Design review of the part built by this model. Coordinates are the model's own, in mm. A direction names the side the tool comes from. Round coordinates to 2 decimals unless told otherwise and drop trailing zeros. Order: outer loops, then holes, each group sorted by start corner. A loop starts at its lowest first (then second) coordinate and runs counter-clockwise, first axis right, second up. Notation, with made-up numbers: (36, 25) - (51, 25) arc R25 cw to (51, 49) - close; hole circle Ø9 at (56.25, 50.5). An arc over 180 degrees is marked (long way). Answer as a JSON object with one key per item and string values. Group by question number.
from build123d import *

# Parameters (mm, degrees)
MODEL_R             = 8
BOSS_EXTRUDE1_DEPTH = 3


with BuildPart() as part:
    # Model → Boss-Extrude1 (new body)
    with BuildSketch(Plane.XY):
        Polygon((11.949818483, 0.880696589), (11.949818483, 30.880698285), (22.949818483, 30.884397455), (22.949818483, 33.884397625), (49.949818483, 33.893477406), (49.949818483, 30.893477236), (60.949818483, 30.897176406), (60.949818483, 0.89717471), (49.949818483, 0.89347554), (49.949818483, -2.10652463), (22.949818483, -2.115604411), (22.949818483, 0.884395759), align=None)
        with Locations((22.949818483, 13.879651404)):
            Circle(MODEL_R, mode=Mode.SUBTRACT)
        with Locations((49.949818483, 13.879651404)):
            Circle(MODEL_R, mode=Mode.SUBTRACT)
    extrude(amount=BOSS_EXTRUDE1_DEPTH)


solid = part.part
1. Mouldability with a two-part tool opening along Y and no side actions: class faces 1 (the cylindrical face through (21.91, 21.81, 1.48)), 2 (the flat face through (11.95, 16, 1)) as pulls with the +Y half, pulls with the -Y half, needs draft (parallel to the pull), parting line crosses it, or undercut.
2. To check wall thickness, follow line 1 (X direction, y = 11.5, z = 1.55); line 2 (X direction, y = 9, z = 0.75); line 3 (Y direction, x = 44, z = 2.25). State the ranges of each line that lie inside material, in increasing order. Write a range as from..to.
3. Take a section at D-D, the plane x = 19. Give the boundary of the cut face in (y, z).
4. Take a section at B-B, the plane x = 51. Give the boundary of the cut face in (y, z), then the cut area to 3 significant figures.
5. Clearance check with flat-ended pins moving along their axes: P1, Ø1, axis at x = 35.5, z = 1, coming from the -Y side; P2, Ø0.9, axis at x = 15, z = 2, coming from the -Y side; P3, Ø1.5, axis at x = 15.5, z = 2, coming from the +Y side. State where each tip first meets the part, or that it passes through.
6. Tool access review of faces 3 (the flat face through (22.95, 32, 1)), 4 (the flat face through (22.95, -1, 1)), 5 (the flat face through (49.95, -1, 1)), 6 (the flat face through (37, 16, 0)), 7 (the flat face through (49.95, 32, 1)): name each direction out of +Z, -Z, +X, -X, +Y, -Y from which nothing blocks a thin tool from reaching the whole face with its end or side.
7. Take a section at A-A, the plane y = 11. Give the boundary of the cut face in (x, z), then the cut area to 3 significant figures.
8. Take a section at C-C, the plane z = 2.1. Give the boundary of the cut face in (x, y).
Response values:
{
 "1": {"face 1": "undercut", "face 2": "needs draft"},
 "2": {"line 1": "11.95..15.31, 30.59..42.31, 57.59..60.95", "line 2": "11.95..16.61, 29.29..43.61, 56.29..60.95", "line 3": "-2.11..8.53, 19.23..33.89"},
 "3": {"outline": "(0.88, 0) - (6.92, 0) - (6.92, 3) - (0.88, 3) - close; (20.84, 0) - (30.88, 0) - (30.88, 3) - (20.84, 3) - close"},
 "4": {"outline": "(0.89, 0) - (5.95, 0) - (5.95, 3) - (0.89, 3) - close; (21.81, 0) - (30.89, 0) - (30.89, 3) - (21.81, 3) - close", "area": "42.4 mm2"},
 "5": {"P1": "y = -2.11", "P2": "y = 0.88", "P3": "y = 30.88"},
 "6": {"face 3": "+Z, -Z, -X, +Y", "face 4": "+Z, -Z, -X, -Y", "face 5": "+Z, -Z, +X, -Y", "face 6": "-Z, +X, -X, +Y, -Y", "face 7": "+Z, -Z, +X, +Y"},
 "7": {"outline": "(11.95, 0) - (15.49, 0) - (15.49, 3) - (11.95, 3) - close; (30.41, 0) - (42.49, 0) - (42.49, 3) - (30.41, 3) - close; (57.41, 0) - (60.95, 0) - (60.95, 3) - (57.41, 3) - close", "area": "57.4 mm2"},
 "8": {"outline": "(11.95, 0.88) - (22.95, 0.88) - (22.95, -2.12) - (49.95, -2.11) - (49.95, 0.89) - (60.95, 0.9) - (60.95, 30.9) - (49.95, 30.89) - (49.95, 33.89) - (22.95, 33.88) - (22.95, 30.88) - (11.95, 30.88) - close; hole circle Ø16 at (22.95, 13.88); hole circle Ø16 at (49.95, 13.88)"}
}
